```python
from build123d import *

# Parameters (mm, degrees)
EXTRUDE001_START = 4
SKETCH002_R      = 3
EXTRUDE001_DEPTH = 3.5
SKETCH001_R      = 1.25
EXTRUDE_DEPTH    = 10


with BuildPart() as extrude001:
    # Sketch002 → Extrude001 (new body)
    with BuildSketch(Plane.XZ.offset(EXTRUDE001_START)):
        with Locations((0, 18.25)):
            Circle(SKETCH002_R)
    extrude(amount=EXTRUDE001_DEPTH)


with BuildPart() as fusion:
    # Sketch001 → Extrude (new body)
    with BuildSketch(Plane.XZ):
        with Locations((0, 18.25)):
            Circle(SKETCH001_R)
    extrude(amount=EXTRUDE_DEPTH)

    # Fusion: union Extrude001
    add(extrude001.part)


with BuildPart() as nya:
    # Sketch → Revolve (revolve)
    with BuildSketch(Plane.XZ):
        with BuildLine():
            Line((2.5, 7), (2.5, 26))
            ThreePointArc((2.5, 26), (2.353553, 26.353553), (2, 26.5))
            Line((0, 26.5), (2, 26.5))
            Line((0, 31), (0, 26.5))
            Line((0, 31), (11.25, 31))
            Line((11.25, 31), (11.25, 27))
            ThreePointArc((11.25, 27), (8.59835, 25.90165), (7.5, 23.25))
            Line((7.5, 23.25), (7.5, 13.25))
            ThreePointArc((7.5, 13.25), (8.59835, 10.59835), (11.25, 9.5))
            Line((11.25, 7), (11.25, 9.5))
            Line((2.5, 7), (11.25, 7))
        make_face()
    revolve(axis=Axis((0, 0, 0), (0, 0, 1)))

    # Cut: cut Fusion
    add(fusion.part, mode=Mode.SUBTRACT)


solid = nya.part
```
Model file for the job. Use its own axes, mm. A direction names the side the tool comes from. Coordinates: 2 decimals unless noted, no trailing zeros. Order: outer loops, then holes, each group sorted by start corner. A loop starts at its lowest first (then second) coordinate and runs counter-clockwise, first axis right, second up. Notation, with made-up numbers: M -24,5.5 L 19,5.5 A29 cw 19,29.5 Z; hole C 40,37 d7. An arc over 180 degrees is marked long. Answer as CSV lines item,"result".
(1) Wall check: line 1 along Z through (x, y) = (0, -3); line 2 along Y through (x, z) = (-2, 24.5); line 3 along Z through (x, y) = (0.5, 8.25). Give the ranges that are in metal, low to high.
Geometry says:
line 1,"z = 7 to 17, 19.5 to 31"
line 2,"y = -7.45 to -1.5, 1.5 to 7.45"
line 3,"z = 7 to 10.98, 25.52 to 31"
(2) 3-axis set-ups, long thin cutter, end or side, ignore diameter. For faces 1 (the cylindrical face through (2.77, -5.73, 17.1)), 2 (the cylindrical face through (5.19, -9.98, 28.97)), 3 (the flat face through (0, 3, 7)), 4 (the flat face through (0, 0, 26.5)), 5 (the cylindrical face through (-0.976, 7.436, 18.18)): which of +Z, -Z, +X, -X, +Y, -Y reach the whole face in a straight line?
Geometry says:
face 1,"-Y"
face 2,"+Z, -Z"
face 3,"-Z, +X, -X, +Y, -Y"
face 4,"-Z"
face 5,"none"
(3) Band-saw the part on B-B, the plane z = 12. List the corners of the cut face in (x, y).
Geometry says:
outline,"C 0,0 d15.43; hole C 0,0 d5"
(4) Band-saw the part on C-C, the plane z = 18.25. List the corners of the cut face in (x, y), then the cut area to 3 significant figures.
Geometry says:
outline,"M -3,-6.87 L -3,-4 L -1.25,-4 L -1.25,-2.17 A2.5 cw long 1.25,-2.17 L 1.25,-4 L 3,-4 L 3,-6.87 A7.5 ccw long Z"
area,"133 mm2"
(5) Pull direction X, two halves, no side cores. Call faces 6 (the cylindrical face through (1.34, 2.11, 16.63)), 7 (the flat face through (0, 0, 31)), 8 (the cylindrical face through (5.19, -9.98, 8.27)): +X half, -X half, draft (parallel to the pull), parting line (faces both ways), or undercut.
Geometry says:
face 6,"undercut"
face 7,"draft"
face 8,"parting line"
(6) Band-saw the part on D-D, the plane z = 23.75. List the corners of the cut face in (x, y).
Geometry says:
outline,"C 0,0 d15.07; hole C 0,0 d5"
(7) Flat gauge pins, fed straight in: pin 1 (1.8 mm diameter, centred on x = 0.5, z = 19.5, fed in from -Y); pin 2 (3 mm diameter, centred on x = -2, z = 21, fed in from +Y); pin 3 (5 mm diameter, centred on y = 9, z = 23.5, fed in from -X). Where does each tip first touch, or does it go through?
Geometry says:
pin 1,"stops at y = -4"
pin 2,"stops at y = 7.48"
pin 3,"stops at x = -3.81"
(8) Band-saw the part on A-A, the plane x = 0. List the corners of the cut face in (y, z).
Geometry says:
outline,"M -11.25,7 L -2.5,7 L -2.5,17 L -4,17 L -4,15.25 L -7.5,15.25 L -7.5,13.25 A3.75 cw -11.25,9.5 Z; M -11.25,27 A3.75 cw -7.5,23.25 L -7.5,21.25 L -4,21.25 L -4,19.5 L -2.5,19.5 L -2.5,26 A0.5 cw -2,26.5 L 2,26.5 A0.5 cw 2.5,26 L 2.5,7 L 11.25,7 L 11.25,9.5 A3.75 cw 7.5,13.25 L 7.5,23.25 A3.75 cw 11.25,27 L 11.25,31 L -11.25,31 Z"
